Verification items for the finished model (mm, model axes). A direction names the side the tool comes from. Round coordinates to 2 decimals unless told otherwise and drop trailing zeros. Loops run counter-clockwise (first coordinate to the right, second up) from the corner with the lowest first, then second, coordinate; pieces in that order, holes last. Notation, with made-up numbers: M 15.5,-34 L 54.5,-34 A17 ccw 54.5,-15 Z; hole C -29.75,-7.5 d5. An arc over 180 degrees is marked long. One line per item, written item: value.
Autodesk Inventor part; units mm, degrees
ref_plane "YZ Plane" through (0, 0, 0) normal (1, 0, 0) x (0, 1, 0)
ref_plane "XZ Plane" through (0, 0, 0) normal (0, 1, 0) x (-1, 0, 0)
ref_plane "XY Plane" through (0, 0, 0) normal (0, 0, 1) x (1, 0, 0)
sketch "Sketch1" plane through (0, 0, 0) normal (0, 1, 0) x (-1, 0, 0)
  circle A0 centre (0, 7) radius 1.75
  circle A1 centre (0, -7) radius 1.75
  line L0 (7, 10) -> (-3, 10)
  line L1 (-3, 10) -> (-3, -10)
  line L2 (-3, -10) -> (7, -10)
  line L3 (7, -10) -> (7, 10)
  line L4 (7, 3.75) -> (-0.3, 3.75)
  line L5 (-0.3, 3.75) -> (-0.3, -3.75)
  line L6 (-0.3, -3.75) -> (7, -3.75)
  line L7 (7, -3.75) -> (7, 3.75)
  point P0 (0, 0)
  dimension "d0" = 3.5
  dimension "d1" = 3.5
  dimension "d2" = 0
  dimension "d3" = 0
  dimension "d4" = 14
  dimension "d5" = 7
  dimension "d6" = 3
  dimension "d7" = 3
  dimension "d8" = 3
  dimension "d9" = 10
  dimension "d10" = 7.5
  dimension "d11" = 3.75
  dimension "d12" = 0.3
extrude "Extrusion1" add sketch "Sketch1" along normal blind 2 contours L3 L4 L5 L6 L2 L1 L0
ref_plane "Work Plane1" through (0.3, 2, -3.75) normal (0.5, 0.866, 0) x (0, 0, 1)
sketch "Sketch2" plane through (0.3, 2, -3.75) normal (0.5, 0.866, 0) x (0, 0, 1)
  line L0 (0, 0) -> (7.5, 0)
  circle A0 centre (3.75, 0) radius 3.75
  point P0 (3.75, 0.7402)
  dimension "d16" = 7.5
extrude "Extrusion2" cut sketch "Sketch2" along normal through all both and the other way through all
sketch "Sketch3" plane through (0.3, 2, -3.75) normal (0.5, 0.866, 0) x (0, 0, 1)
  circle A0 centre (3.75, 0.7402) radius 3.75
  circle A1 centre (3.75, 0.7402) radius 5
  line L0 (8.75, 0.7402) -> (-1.25, 0.7402)
  point P0 (7.5, 0.7402)
  point P1 (0, 0.7402)
  dimension "d19" = 7.5
  dimension "d20" = 10
extrude "Extrusion3" add sketch "Sketch3" along normal mid plane 10 contours L0 A1 A0 picked at (8.2486, 0.0422)
sketch "Sketch4" plane through (-7, 0, -10) normal (-1, 0, 0) x (0, 0, 1)
  line L0 (6.25, 0) -> (5, 0)
  line L1 (12.9317, 2) -> (13.7317, 2)
  line L2 (6.25, 0) -> (13.7317, 0)
  line L3 (13.7317, 0) -> (13.7317, 2)
  line L4 (13.7317, 2) -> (6.25, 2)
  line L5 (6.25, 2) -> (6.25, 0)
  point P0 (10, 0)
  point P1 (12.9317, 2)
extrude "Extrusion4" add sketch "Sketch4" against normal blind 5
sketch "Sketch5" plane through (-7, 0, 10) normal (0, 0, 1) x (1, 0, 0)
  line L0 (0, 0) -> (0, 2)
  line L1 (0, 0) -> (10, 0)
  line L2 (10, 0) -> (10, -5)
  line L3 (10, -5) -> (0, -5)
  line L4 (0, -5) -> (0, 0)
  point P0 (7, 0)
  dimension "d25" = 10
  dimension "d26" = 5
extrude "Extrusion5" cut sketch "Sketch5" against normal through all
sketch "Sketch6" plane through (0.3, 2, -3.75) normal (0.5, 0.866, 0) x (0, 0, 1)
  circle A0 centre (3.75, 0.7402) radius 3.55
  dimension "d29" = 7.1
extrude "Extrusion6" cut sketch "Sketch6" against normal through all
sketch "Sketch7" plane through (0, 0, 0) normal (0, -1, 0) x (1, 0, 0)
  ellipse E0 centre (0, 0) end of major axis (-4.3301, 0) minor radius 3.75 (0, 3.75) -> (0, -3.75) ccw
  line L0 (3, -2.9317) -> (3, -10)
  line L1 (0, 3.75) -> (3, 3.75)
  line L2 (3, 3.75) -> (3, -3.75)
  line L3 (3, -3.75) -> (0, -3.75)
  line L4 (0, -3.75) -> (0, 3.75)
  point P0 (0, 0)
  dimension "d32" = 7.5
extrude "Extrusion7" cut sketch "Sketch7" against normal up to surface (2 mm away) contours L1 L2 L0 L3 L4
properties part number "Front Bracket"
(1) Sectioned sample at B-B on x = 0.5. Count the separate pieces of the cut face and the enclosed holes in it, and give its area (3 significant figures).
Completed:
separate pieces: 4
enclosed holes: 0
area: 28.3 mm^2
(2) Sectioned sample at C-C on z = 0.5. Enter the section's corners in (x, y).
Completed:
outline: M -7,0 L -4.06,0 L -2.9,2 L -3.14,2 L 0.22,7.82 L -0.87,8.45 L -4.59,2 L -7,2 Z
(3) Tool access check on faces 1 (the face through (2, 1, -3.75)), 2 (the face through (-2, 1, -10)), 3 (the face through (3, 1, -7)), 4 (the face through (2.28, 3.95, 4.38)). Record the directions out of +Z, -Z, +X, -X, +Y, -Y that give a thin tool (end or side, any length) a straight path to the whole face; none if there is none.
Completed:
face 1: +X, -Y
face 2: -Z, +X, -X, +Y, -Y
face 3: +Z, -Z, +X, -Y
face 4: +Z, -Z, +X
(4) Mould release check, pull along X, two halves, no side actions. Record for faces 5 (the face through (-1.366, 5.132, 0.082)), 6 (the face through (-2, 1, 10)), 7 (the face through (0.38, 0.99, -5.29)): +X half, -X half, draft (parallel to the pull), parting line (faces both ways), or undercut.
Completed:
face 5: +X half
face 6: draft
face 7: undercut
(5) Sectioned sample at A-A on z = 7. Enter the section's corners in (x, y).
Completed:
outline: M -7,0 L -1.75,0 L -1.75,2 L -7,2 Z; M 1.75,0 L 3,0 L 3,2 L 1.75,2 Z
(6) Sectioned sample at D-D on z = -7.5. Enter the section's corners in (x, y), and give its area (3 significant figures).
Completed:
outline: M -7,0 L -1.68,0 L -1.68,2 L -7,2 Z; M 1.68,0 L 3,0 L 3,2 L 1.68,2 Z
area: 13.3 mm^2
(7) Depth check by flat-ended pin: pin 1 Ø5 at (x, z) = (-3, -4.5) entering from +Y; pin 2 Ø0.6 at (x, z) = (-2.5, -0.5) entering from +Y; pin 3 Ø2 at (y, z) = (1, -7.5) entering from +X. Enter the tip coordinate at first touch or a pass-through.
Completed:
pin 1: stops at y = 6.28
pin 2: stops at y = 6.14
pin 3: stops at x = 3
